Model file for the job. Use its own axes, mm. Face numbers are marked on the shaded views. A direction names the side the tool comes from. Coordinates: 2 decimals unless noted, no trailing zeros. Order: outer loops, then holes, each group sorted by start corner. A loop starts at its lowest first (then second) coordinate and runs counter-clockwise, first axis right, second up. Notation, with made-up numbers: (19.5, 14) -> (29.5, 14) arc R14 cw to (29.5, 27) -> close; hole circle Ø8 at (67, 61.5). An arc over 180 degrees is marked (long way). Return JSON: item names as keys, results as strings. Group by question number.
1) Cut at D-D (z = -23.5). Write the cut outline in (x, y).
2) Which spindle directions (+Z, -Z, +X, -X, +Y, -Y) get a long thin tool onto all of the face, cutting with end or side? Do the marked faces 1 and 2. Say none if no direction does.
3) Cut at A-A (z = 0). Write the cut outline in (x, y).
4) Cut at B-B (x = 0). Write the cut outline in (y, z).
5) Flat gauge pins, fed straight in: pin 1 (2 mm diameter, centred on y = 6.5, z = -31.5, fed in from -X); pin 2 (3 mm diameter, centred on x = -55, y = 7, fed in from +Z); pin 3 (2 mm diameter, centred on y = 4, z = -40, fed in from -X). Where does each tip first touch, or does it go through?
6) Cut at C-C (y = 7). Write the cut outline in (x, z), and give its area (3 significant figures).
7) Pull direction X, two halves, no side cores. Call the marked faces 3, 4 and 5: +X half, -X half, draft (parallel to the pull), parting line (faces both ways), or undercut.
8) Probe line 1 (X direction, y = 1, z = 2); line 2 (X direction, y = 11.5, z = 23.5); line 3 (Z direction, x = 29, y = 8.5). List the from-to ranges inside material, lowest first.
from build123d import *

# Parameters (mm, degrees)
SKETCH1_R           = 87.5
BOSS_EXTRUDE1_DEPTH = 16
SKETCH2_R           = 27.5
CUT_EXTRUDE1_DEPTH  = 125.773795326
SKETCH3_R           = 7.307789365
CUT_EXTRUDE2_DEPTH  = 13.99423
CIRPATTERN1_START   = 2.005769827
CIRPATTERN1_DEPTH   = 13.994230173


# Read off the part's stored shape, not the designer's step: CirPattern1
with BuildPart() as part:
    # Sketch1 → Boss-Extrude1 (new body)
    with BuildSketch(Plane(origin=(0, 0, 0), x_dir=(1, 0, 0), z_dir=(0, 1, 0))):
        with Locations(Location((0, 0, 0), (0, 0, 270))):
            Circle(SKETCH1_R)
    extrude(amount=BOSS_EXTRUDE1_DEPTH)

    # Sketch2 → Cut-Extrude1 (cut, through all)
    with BuildSketch(Plane(origin=(0, 0, 0), x_dir=(1, 0, 0), z_dir=(0, 1, 0))):
        with Locations(Location((0, 0, 0), (0, 0, 270))):
            Circle(SKETCH2_R)
    extrude(amount=CUT_EXTRUDE1_DEPTH, mode=Mode.SUBTRACT)

    # Sketch3 → Cut-Extrude2 (cut)
    with BuildSketch(Plane(origin=(0, 16, 0), x_dir=(1, 0, 0), z_dir=(0, 1, 0))):
        with Locations((-34.289217919, 0)):
            Circle(SKETCH3_R)
    extrude(amount=-CUT_EXTRUDE2_DEPTH, mode=Mode.SUBTRACT)

    # CirPattern1 outline → CirPattern1 (cut)
    with BuildSketch(Plane(origin=(0, 0, 0), x_dir=(1, 0, 0), z_dir=(0, 1, 0)).offset(CIRPATTERN1_START)):
        with BuildLine():
            ThreePointArc((-17.65957637, -21.080544643), (-19.445436483, -19.445436483), (-21.080544643, -17.65957637))
            ThreePointArc((-21.080544643, -17.65957637), (-29.413525928, -29.413525928), (-17.65957637, -21.080544643))
        make_face()
        with BuildLine():
            ThreePointArc((-17.65957637, 21.080544643), (-29.413525928, 29.413525928), (-21.080544643, 17.65957637))
            ThreePointArc((-21.080544643, 17.65957637), (-19.445436483, 19.445436483), (-17.65957637, 21.080544643))
        make_face()
        with BuildLine():
            ThreePointArc((2.418989864, -27.393402272), (0, -27.5), (-2.418989864, -27.393402272))
            ThreePointArc((-2.418989864, -27.393402272), (0, -41.597007284), (2.418989864, -27.393402272))
        make_face()
        with BuildLine():
            ThreePointArc((2.418989864, 27.393402272), (0, 41.597007284), (-2.418989864, 27.393402272))
            ThreePointArc((-2.418989864, 27.393402272), (0, 27.5), (2.418989864, 27.393402272))
        make_face()
        with BuildLine():
            ThreePointArc((21.080544643, -17.65957637), (19.445436483, -19.445436483), (17.65957637, -21.080544643))
            ThreePointArc((17.65957637, -21.080544643), (29.413525928, -29.413525928), (21.080544643, -17.65957637))
        make_face()
        with BuildLine():
            ThreePointArc((21.080544643, 17.65957637), (29.413525928, 29.413525928), (17.65957637, 21.080544643))
            ThreePointArc((17.65957637, 21.080544643), (19.445436483, 19.445436483), (21.080544643, 17.65957637))
        make_face()
        with BuildLine():
            ThreePointArc((27.393402272, 2.418989864), (27.5, 0), (27.393402272, -2.418989864))
            ThreePointArc((27.393402272, -2.418989864), (41.597007284, 0), (27.393402272, 2.418989864))
        make_face()
    extrude(amount=CIRPATTERN1_DEPTH, mode=Mode.SUBTRACT)


solid = part.part
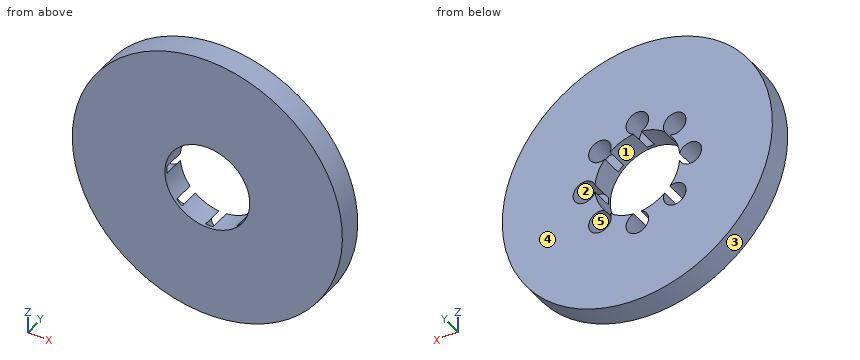
Answers below:
{
 "1": {"outline": "(-84.29, 0) -> (-14.28, 0) -> (-14.28, 16) -> (-16.98, 16) -> (-16.98, 2.01) -> (-31.52, 2.01) -> (-31.52, 16) -> (-84.29, 16) -> close; (14.28, 0) -> (84.29, 0) -> (84.29, 16) -> (31.52, 16) -> (31.52, 2.01) -> (16.98, 2.01) -> (16.98, 16) -> (14.28, 16) -> close"},
 "2": {"face 1": "+Y, -Y", "face 2": "+Y"},
 "3": {"outline": "(-87.5, 0) -> (-27.5, 0) -> (-27.5, 2.01) -> (-41.6, 2.01) -> (-41.6, 16) -> (-87.5, 16) -> close; (27.5, 0) -> (87.5, 0) -> (87.5, 16) -> (41.6, 16) -> (41.6, 2.01) -> (27.5, 2.01) -> close"},
 "4": {"outline": "(0, -87.5) -> (16, -87.5) -> (16, -41.6) -> (2.01, -41.6) -> (2.01, -27.5) -> (0, -27.5) -> close; (0, 27.5) -> (2.01, 27.5) -> (2.01, 41.6) -> (16, 41.6) -> (16, 87.5) -> (0, 87.5) -> close"},
 "5": {"pin 1": "stops at x = -82.01", "pin 2": "stops at z = 69.24", "pin 3": "stops at x = -78.33"},
 "6": {"outline": "circle Ø175 at (0, 0); hole (-27.39, -2.42) arc R27.5 ccw to (-21.08, -17.66) arc R7.31 ccw (long way) to (-17.66, -21.08) arc R27.5 ccw to (-2.42, -27.39) arc R7.31 ccw (long way) to (2.42, -27.39) arc R27.5 ccw to (17.66, -21.08) arc R7.31 ccw (long way) to (21.08, -17.66) arc R27.5 ccw to (27.39, -2.42) arc R7.31 ccw (long way) to (27.39, 2.42) arc R27.5 ccw to (21.08, 17.66) arc R7.31 ccw (long way) to (17.66, 21.08) arc R27.5 ccw to (2.42, 27.39) arc R7.31 ccw (long way) to (-2.42, 27.39) arc R27.5 ccw to (-17.66, 21.08) arc R7.31 ccw (long way) to (-21.08, 17.66) arc R27.5 ccw to (-27.39, 2.42) arc R7.31 ccw (long way) to start", "area": "20,300 mm^2"},
 "7": {"face 3": "parting line", "face 4": "draft", "face 5": "undercut"},
 "8": {"line 1": "x = -87.48 to -27.43, 27.43 to 87.48", "line 2": "x = -84.29 to -31.52, -16.98 to -14.28, 14.28 to 16.98, 31.52 to 84.29", "line 3": "z = -82.55 to -29.8, -18.7 to -5.04, 5.04 to 18.7, 29.8 to 82.55"}
}
